The listing builds one solid part. Answer for the finished solid, in the listing's coordinates (mm). Face numbers are marked on the shaded views. Coordinates: 2 decimals unless noted, no trailing zeros. Write each loop counter-clockwise with the first axis right and the second up, starting at its lowest first coordinate (ties: lowest second). Pieces come first, ordered by that corner, then holes. Notation, with made-up numbers: M -22,5.5 L 13,5.5 A16 cw 13,19.5 Z; hole C -17,-11.75 d8. An arc over 180 degrees is marked long. Put each result on its own line as item: value. Start each with the question number.
```python
from build123d import *

# Parameters (mm, degrees)
F0_R        = 10.5
F0_R_2      = 9.7
F1_DEPTH    = 44
F3_DEPTH    = 20.75
F4_T1_DEPTH = 10.8988435946
F4_T3_DEPTH = 10.8988435946
F5_R        = 0.3
F6_R        = 1


# Not quite as in the source:
# - a fillet or chamfer that OpenCascade refuses, or shapes differently, is made with other operations: its cross-section is extruded or revolved along the edge and cut away or added


with BuildPart() as f1:
    # F0 (on Top) → F1 (new body)
    with BuildSketch(Plane.XY):
        Circle(F0_R)
        Circle(F0_R_2, mode=Mode.SUBTRACT)
    extrude(amount=F1_DEPTH)

    # F2 (on Right) → F3 (cut, symmetric)
    with BuildSketch(Plane.YZ):
        Polygon((-11.3, 0), (-11.3, -7.5), (11.3, -7.5), (11.3, 0), (4.6, 0), (4.6, 13), (-4.6, 13), (-4.6, 0), align=None)
    extrude(amount=F3_DEPTH, both=True, mode=Mode.SUBTRACT)

    # F4: fillet of radius 2 on 4 edges, made by hand

    # F4_s2 → F4_t1 (cut)
    with BuildSketch(Plane.YZ.offset(-14.4387499172)):
        with BuildLine():
            ThreePointArc((-4.6, 2), (-5.1857864376, 0.5857864376), (-6.6, 0))
            Line((-6.6, 0), (-4.6, 0))
            Line((-4.6, 0), (-4.6, 2))
        make_face()
        with BuildLine():
            ThreePointArc((6.6, 0), (5.1857864376, 0.5857864376), (4.6, 2))
            Line((4.6, 2), (4.6, 0))
            Line((4.6, 0), (6.6, 0))
        make_face()
    extrude(amount=F4_T1_DEPTH, mode=Mode.SUBTRACT)

    # F4_s4 → F4_t3 (cut)
    with BuildSketch(Plane.YZ.offset(3.5399063227)):
        with BuildLine():
            ThreePointArc((-6.6, 0), (-5.1857864376, 0.5857864376), (-4.6, 2))
            Line((-4.6, 2), (-4.6, 0))
            Line((-4.6, 0), (-6.6, 0))
        make_face()
        with BuildLine():
            ThreePointArc((4.6, 2), (5.1857864376, 0.5857864376), (6.6, 0))
            Line((6.6, 0), (4.6, 0))
            Line((4.6, 0), (4.6, 2))
        make_face()
    extrude(amount=F4_T3_DEPTH, mode=Mode.SUBTRACT)

    # F5
    f5_edges = [f1.edges().sort_by_distance(p)[0] for p in [
        (-10.5, 0, 44),
        (-9.7, 0, 44),
    ]]
    fillet(f5_edges, radius=F5_R)

    # F6
    f6_edges = [f1.edges().sort_by_distance(p)[0] for p in [
        (8.989328, -4.6, 13),
        (-8.989328, -4.6, 13),
        (8.989328, 4.6, 13),
        (-8.989328, 4.6, 13),
    ]]
    fillet(f6_edges, radius=F6_R)


solid = f1.part
```
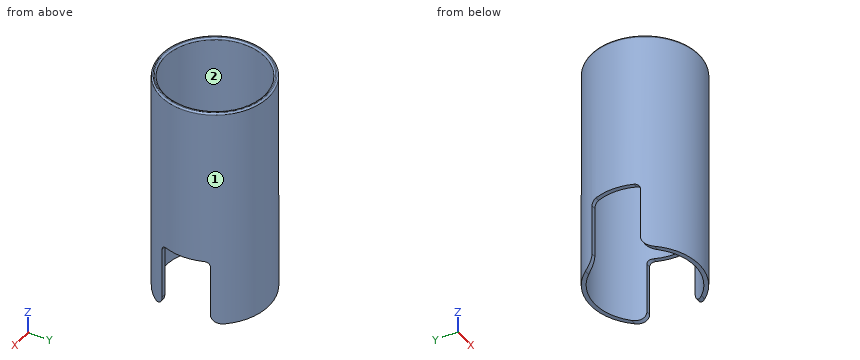
1) A cutting plane is placed at D-D on z = 15.5. Write down the section's boundary in (x, y), then the cut area to 3 significant figures.
2) A cutting plane is placed at A-A on y = 0. Write down the section's boundary in (x, z).
3) Determine the mould class of the marked faces 1 and 2 for opening direction Y: +Y half, -Y half, draft (parallel to the pull), parting line (faces both ways), or undercut.
4) A cutting plane is placed at C-C on x = 0. Write down the section's boundary in (y, z), then the cut area to 3 significant figures.
5) A cutting plane is placed at B-B on z = 7.5. Write down the section's boundary in (x, y).
6) Given pin 1 Ø12 at (y, z) = (-7.5, 25.5) entering from +X; pin 2 Ø1 at (x, z) = (9, 8) entering from +Y; pin 3 Ø8 at (x, y) = (-2.5, 2) entering from +Z; pin 4 Ø2 at (y, z) = (-5.5, 9) entering from +X, each flat-ended and moving along its own axis, determine where each tip first touches the part or whether it passes through.
7) Straight lines are drawn through the part: probe 1 along Y at (x, z) = (0, 33); probe 2 along Y at (x, z) = (-6.75, 10); probe 3 along X at (y, z) = (6, 11). For each, find the intervals that lie inside material, in ascending order.
Answers follow:
1. outline: C 0,0 d21; hole C 0,0 d19.4
1. area: 50.8 mm²
2. outline: M -10.5,13 L -9.7,13 L -9.7,43.7 A0.3 ccw -10,44 L -10.2,44 A0.3 ccw -10.5,43.7 Z; M 9.7,13 L 10.5,13 L 10.5,43.7 A0.3 ccw 10.2,44 L 10,44 A0.3 ccw 9.7,43.7 Z
3. face 1: parting line
3. face 2: undercut
4. outline: M -10.5,0 L -9.7,0 L -9.7,43.7 A0.3 ccw -10,44 L -10.2,44 A0.3 ccw -10.5,43.7 Z; M 9.7,0 L 10.5,0 L 10.5,43.7 A0.3 ccw 10.2,44 L 10,44 A0.3 ccw 9.7,43.7 Z
4. area: 70.3 mm²
5. outline: M -9.44,-4.6 A10.5 ccw 9.44,-4.6 L 8.54,-4.6 A9.7 cw -8.54,-4.6 Z; M -9.44,4.6 L -8.54,4.6 A9.7 cw 8.54,4.6 L 9.44,4.6 A10.5 ccw Z
6. pin 1: stops at x = 10.39
6. pin 2: stops at y = 6.16
6. pin 3: passes through
6. pin 4: stops at x = 9.44
7. probe 1: y = -10.5 to -9.7, 9.7 to 10.5
7. probe 2: y = -8.04 to -6.97, 6.97 to 8.04
7. probe 3: x = -8.62 to -7.62, 7.62 to 8.62
